from build123d import *

# Parameters (mm, degrees)
SKIZZE1_W                       = 25
SKIZZE1_H                       = 25
AUFSATZ_LINEAR_AUSTRAGEN1_DEPTH = 2
SKIZZE2_W                       = 21.7
SKIZZE2_H                       = 21.7
SKIZZE2_W_2                     = 17.7
SKIZZE2_H_2                     = 17.7
LINEAR_AUSTRAGEN_D_NN1_DEPTH    = 5
VERRUNDUNG1_R                   = 1
LINEAR_AUSTRAGEN_D_NN2_DEPTH    = 2
FASE1_SIZE                      = 0.75
FASE1_SIZE2                     = 1.299038106
VERRUNDUNG2_R                   = 0.5
VERRUNDUNG3_R                   = 1
FASE2_SIZE                      = 1
VERRUNDUNG5_R                   = 0.5
VERRUNDUNG4_R                   = 0.5
VERRUNDUNG6_R                   = 1


with BuildPart() as part:
    # Skizze1 → Aufsatz-Linear austragen1 (new body)
    with BuildSketch(Plane.XY):
        Rectangle(SKIZZE1_W, SKIZZE1_H)
    extrude(amount=AUFSATZ_LINEAR_AUSTRAGEN1_DEPTH)

    # Skizze2 → Linear-Austragen-Dünn1 (add)
    with BuildSketch(Plane.XY.offset(2)):
        Rectangle(SKIZZE2_W, SKIZZE2_H)
        Rectangle(SKIZZE2_W_2, SKIZZE2_H_2, mode=Mode.SUBTRACT)
    extrude(amount=LINEAR_AUSTRAGEN_D_NN1_DEPTH)

    # Verrundung1
    verrundung1_edges = [part.edges().sort_by_distance(p)[0] for p in [
        (-10.85, -10.85, 4.5),
        (10.85, -10.85, 4.5),
        (10.85, 10.85, 4.5),
        (-10.85, 10.85, 4.5),
    ]]
    fillet(verrundung1_edges, radius=VERRUNDUNG1_R)

    # Skizze3 → Linear-Austragen-Dünn2 (add)
    with BuildSketch(Plane.XY.offset(7)):
        with BuildLine():
            Line((9.85, 11.1), (-9.85, 11.1))
            ThreePointArc((-9.85, 11.1), (-10.733883476, 10.733883476), (-11.1, 9.85))
            Line((-11.1, 9.85), (-11.1, -9.85))
            ThreePointArc((-11.1, -9.85), (-10.733883476, -10.733883476), (-9.85, -11.1))
            Line((-9.85, -11.1), (9.85, -11.1))
            ThreePointArc((9.85, -11.1), (10.733883476, -10.733883476), (11.1, -9.85))
            Line((11.1, -9.85), (11.1, 9.85))
            ThreePointArc((11.1, 9.85), (10.733883476, 10.733883476), (9.85, 11.1))
        make_face()
        with BuildLine():
            Line((9.85, 10.85), (-9.85, 10.85))
            ThreePointArc((-9.85, 10.85), (-10.557106781, 10.557106781), (-10.85, 9.85))
            Line((-10.85, 9.85), (-10.85, -9.85))
            ThreePointArc((-10.85, -9.85), (-10.557106781, -10.557106781), (-9.85, -10.85))
            Line((-9.85, -10.85), (9.85, -10.85))
            ThreePointArc((9.85, -10.85), (10.557106781, -10.557106781), (10.85, -9.85))
            Line((10.85, -9.85), (10.85, 9.85))
            ThreePointArc((10.85, 9.85), (10.557106781, 10.557106781), (9.85, 10.85))
        make_face(mode=Mode.SUBTRACT)
    extrude(amount=-LINEAR_AUSTRAGEN_D_NN2_DEPTH)

    # Fase1
    fase1_edges = [part.edges().sort_by_distance(p)[0] for p in [
        (10.733883476, 10.733883476, 7),
        (0, 11.1, 7),
        (-10.733883476, 10.733883476, 7),
        (-11.1, 0, 7),
        (-10.733883476, -10.733883476, 7),
        (0, -11.1, 7),
        (10.733883476, -10.733883476, 7),
        (11.1, 0, 7),
    ]]
    fase1_side = [part.faces().sort_by_distance(p)[0] for p in [
        (10.511883476, 10.511883476, 7),
    ]]
    chamfer(fase1_edges, length=FASE1_SIZE, length2=FASE1_SIZE2, reference=fase1_side[0])

    # Verrundung2
    # the kernel refuses this fillet: 0.5 mm, written as the material it adds along each edge
    with BuildSketch(Plane(origin=(10.85, -9.85, 5), x_dir=(1, 0, 0), z_dir=(0, 1, 0)), Plane(origin=(9.85, 10.85, 5), x_dir=(0, 1, 0), z_dir=(-1, 0, 0)), Plane(origin=(-10.85, 9.85, 5), x_dir=(-1, 0, 0), z_dir=(0, -1, 0)), Plane(origin=(-9.85, -10.85, 5), x_dir=(0, -1, 0), z_dir=(1, 0, 0))) as verrundung2_piece_1:
        with BuildLine():
            CenterArc((0.5, 0.433012702), VERRUNDUNG2_R, 180, 60)
            Line((0, 0.433012702), (-0.01, 0.433012702))
            Line((-0.01, 0.433012702), (-0.01, 0))
            Line((-0.01, 0), (0, -0.01))
            ThreePointArc((0, -0.01), (0.125, -0.01), (0.245, -0.008660254))
            Line((0.245, -0.008660254), (0.25, 0))
        make_face()
    extrude(amount=19.7)
    with BuildSketch(Plane(origin=(9.85, 9.85, 5), x_dir=(1, 0, 0), z_dir=(0, -1, 0))) as verrundung2_piece_2:
        with BuildLine():
            CenterArc((1.5, -0.433012702), VERRUNDUNG2_R, 120, 60)
            Line((1, -0.433012702), (0.99, -0.433012702))
            Line((0.99, -0.433012702), (0.99, 0))
            Line((0.99, 0), (1, 0.01))
            ThreePointArc((1, 0.01), (1.125, 0.01), (1.245, 0.008660254))
            Line((1.245, 0.008660254), (1.25, 0))
        make_face()
    revolve(axis=Axis((9.85, 9.85, 5), (0, 0, 1)), revolution_arc=90)
    with BuildSketch(Plane(origin=(-9.85, 9.85, 5), x_dir=(0, 1, 0), z_dir=(1, 0, 0))) as verrundung2_piece_3:
        with BuildLine():
            CenterArc((1.5, -0.433012702), VERRUNDUNG2_R, 120, 60)
            Line((1, -0.433012702), (0.99, -0.433012702))
            Line((0.99, -0.433012702), (0.99, 0))
            Line((0.99, 0), (1, 0.01))
            ThreePointArc((1, 0.01), (1.125, 0.01), (1.245, 0.008660254))
            Line((1.245, 0.008660254), (1.25, 0))
        make_face()
    revolve(axis=Axis((-9.85, 9.85, 5), (0, 0, 1)), revolution_arc=90)
    with BuildSketch(Plane(origin=(-9.85, -9.85, 5), x_dir=(-1, 0, 0), z_dir=(0, 1, 0))) as verrundung2_piece_4:
        with BuildLine():
            CenterArc((1.5, -0.433012702), VERRUNDUNG2_R, 120, 60)
            Line((1, -0.433012702), (0.99, -0.433012702))
            Line((0.99, -0.433012702), (0.99, 0))
            Line((0.99, 0), (1, 0.01))
            ThreePointArc((1, 0.01), (1.125, 0.01), (1.245, 0.008660254))
            Line((1.245, 0.008660254), (1.25, 0))
        make_face()
    revolve(axis=Axis((-9.85, -9.85, 5), (0, 0, 1)), revolution_arc=90)
    with BuildSketch(Plane(origin=(9.85, -9.85, 5), x_dir=(0, -1, 0), z_dir=(-1, 0, 0))) as verrundung2_piece_5:
        with BuildLine():
            CenterArc((1.5, -0.433012702), VERRUNDUNG2_R, 120, 60)
            Line((1, -0.433012702), (0.99, -0.433012702))
            Line((0.99, -0.433012702), (0.99, 0))
            Line((0.99, 0), (1, 0.01))
            ThreePointArc((1, 0.01), (1.125, 0.01), (1.245, 0.008660254))
            Line((1.245, 0.008660254), (1.25, 0))
        make_face()
    revolve(axis=Axis((9.85, -9.85, 5), (0, 0, 1)), revolution_arc=90)

    # Verrundung3
    verrundung3_edges = [part.edges().sort_by_distance(p)[0] for p in [
        (0, -11.1, 5.700961894),
        (10.733883476, -10.733883476, 5.700961894),
        (-10.733883476, -10.733883476, 5.700961894),
        (11.1, 0, 5.700961894),
        (-11.1, 0, 5.700961894),
        (10.733883476, 10.733883476, 5.700961894),
        (-10.733883476, 10.733883476, 5.700961894),
        (0, 11.1, 5.700961894),
        (10.733883476, 10.733883476, 5),
        (11.1, 0, 5),
        (10.733883476, -10.733883476, 5),
        (0, -11.1, 5),
        (-10.733883476, -10.733883476, 5),
        (-11.1, 0, 5),
        (-10.733883476, 10.733883476, 5),
        (0, 11.1, 5),
    ]]
    fillet(verrundung3_edges, radius=VERRUNDUNG3_R)

    # Fase2
    fase2_edges = [part.edges().sort_by_distance(p)[0] for p in [
        (0, 12.5, 2),
    ]]
    chamfer(fase2_edges, length=FASE2_SIZE)

    # Verrundung5
    verrundung5_edges = [part.edges().sort_by_distance(p)[0] for p in [
        (0, 12.5, 1),
    ]]
    fillet(verrundung5_edges, radius=VERRUNDUNG5_R)

    # Verrundung4
    verrundung4_edges = [part.edges().sort_by_distance(p)[0] for p in [
        (-12.5, 11.926776695, 1.573223305),
        (-12.5, 12.5, 0.396446609),
        (12.5, 12.5, 0.396446609),
        (12.5, 11.926776695, 1.573223305),
        (12.5, 12.461939766, 0.984234935),
        (-12.5, 12.461939766, 0.984234935),
        (12.5, -12.5, 1),
        (-12.5, -12.5, 1),
    ]]
    fillet(verrundung4_edges, radius=VERRUNDUNG4_R)

    # Verrundung6
    verrundung6_edges = [part.edges().sort_by_distance(p)[0] for p in [
        (0, -8.85, 2),
        (8.85, 0, 2),
        (0, 8.85, 2),
        (-8.85, 0, 2),
        (8.85, -8.85, 4.5),
        (8.85, 8.85, 4.5),
        (-8.85, 8.85, 4.5),
        (-8.85, -8.85, 4.5),
    ]]
    fillet(verrundung6_edges, radius=VERRUNDUNG6_R)


solid = part.part
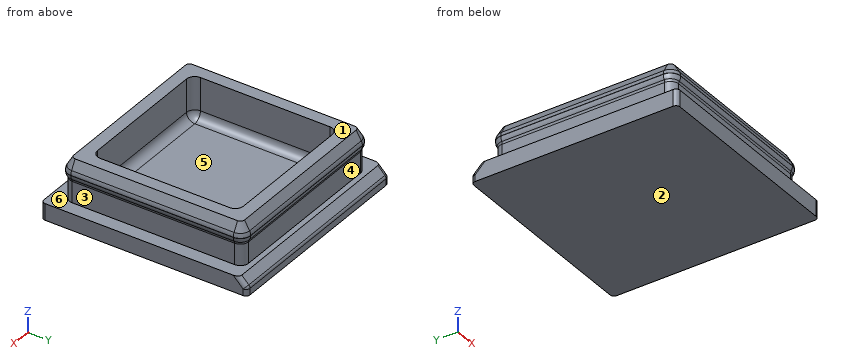
Part model, mm, in its own coordinate system. Face numbers are marked on the shaded views. A direction names the side the tool comes from. Coordinates: 2 decimals unless noted, no trailing zeros. Loops run counter-clockwise (first coordinate to the right, second up) from the corner with the lowest first, then second, coordinate; pieces in that order, holes last. Notation, with made-up numbers: (-26.5, 61) -> (14.5, 61) arc R28 cw to (14.5, 83) -> close; hole circle Ø9 at (-11.5, 14). An arc over 180 degrees is marked (long way). Use a Markdown table: item, result. Add a question column.
Item 1: Probe probe 1 along Y at (x, z) = (7.75, 3.25); probe 2 along Y at (x, z) = (-5, 6). List the from-to ranges inside material, lowest first.
Item 2: Band-saw the part on A-A on z = 4. Write the cut outline in (x, y).
Item 3: Pull direction Z, two halves, no side cores. Call the marked faces 1, 2 and 3: +Z half, -Z half, draft (parallel to the pull), parting line (faces both ways), or undercut.
Item 4: Flat gauge pins, fed straight in: P1, Ø1, axis at y = -2, z = 3.5, coming from the +X side; P2, Ø4.5, axis at x = -2, y = -3, coming from the +Z side; P3, Ø2, axis at y = -2, z = 6, coming from the -X side; P4, Ø12, axis at x = -5.5, y = 3.5, coming from the +Z side. Where does each tip first touch, or does it go through?
Item 5: Which spindle directions (+Z, -Z, +X, -X, +Y, -Y) get a long thin tool onto all of the face, cutting with end or side? Do the marked faces 4, 5 and 6. Say none if no direction does.
Geometry says:
| question | item | result |
|---|---|---|
| 1 | probe 1 | -10.85 to -8.85, 8.85 to 10.85 |
| 1 | probe 2 | -10.93 to -8.85, 8.85 to 10.93 |
| 2 | outline | (-10.85, -9.85) arc R1 ccw to (-9.85, -10.85) -> (9.85, -10.85) arc R1 ccw to (10.85, -9.85) -> (10.85, 9.85) arc R1 ccw to (9.85, 10.85) -> (-9.85, 10.85) arc R1 ccw to (-10.85, 9.85) -> close; hole (-8.85, -7.85) arc R1 ccw to (-7.85, -8.85) -> (7.85, -8.85) arc R1 ccw to (8.85, -7.85) -> (8.85, 7.85) arc R1 ccw to (7.85, 8.85) -> (-7.85, 8.85) arc R1 ccw to (-8.85, 7.85) -> close |
| 3 | face 1 | +Z half |
| 3 | face 2 | -Z half |
| 3 | face 3 | undercut |
| 4 | P1 | x = 10.85 |
| 4 | P2 | z = 2 |
| 4 | P3 | x = -11.1 |
| 4 | P4 | z = 7 |
| 5 | face 4 | +X, -X, +Y |
| 5 | face 5 | +Z |
| 5 | face 6 | none |
